```python
from build123d import *

# Parameters (mm, degrees)
SKIZZE1_W                       = 47.557374535
SKIZZE1_H                       = 4
AUFSATZ_LINEAR_AUSTRAGEN1_DEPTH = 76
AUFSATZ_LINEAR_AUSTRAGEN2_DEPTH = 47.557374535
VERRUNDUNG1_R                   = 10
SKIZZE3_R                       = 3.3
SCHNITT_LINEAR_AUSTRAGEN1_DEPTH = 47.557374535
SKIZZE4_W                       = 47.557374535
SKIZZE4_H                       = 15
SCHNITT_LINEAR_AUSTRAGEN2_DEPTH = 30
SKIZZE5_W                       = 47.557374535
SKIZZE5_H                       = 34.5
TEMPOR_R_DEPTH                  = 20


with BuildPart() as part:
    # Skizze1 → Aufsatz-Linear austragen1 (new body)
    with BuildSketch(Plane.ZY.offset(38)):
        with Locations((46.278687268, -2)):
            Rectangle(SKIZZE1_W, SKIZZE1_H)
    extrude(amount=-AUFSATZ_LINEAR_AUSTRAGEN1_DEPTH)

    # Skizze2 → Aufsatz-Linear austragen2 (add)
    with BuildSketch(Plane.XY.offset(22.5)):
        Polygon((-38, 65), (-38, 0), (-28, 0), (-22.226497308, 10), (-28, 20), (-28, 45), (-22.226497308, 55), (-28, 65), align=None)
        Polygon((28, 65), (38, 65), (38, 0), (28, 0), (22.226497308, 10), (28, 20), (28, 45), (22.226497308, 55), align=None)
    extrude(amount=AUFSATZ_LINEAR_AUSTRAGEN2_DEPTH)

    # Verrundung1
    verrundung1_edges = [part.edges().sort_by_distance(p)[0] for p in [
        (-22.226497308, 10, 46.278687268),
        (-22.226497308, 55, 46.278687268),
        (22.226497308, 55, 46.278687268),
        (22.226497308, 10, 46.278687268),
    ]]
    fillet(verrundung1_edges, radius=VERRUNDUNG1_R)

    # Skizze3 → Schnitt-Linear austragen1 (cut)
    with BuildSketch(Plane(origin=(0, 0, 22.5), x_dir=(-1, 0, 0), z_dir=(0, 0, -1))):
        with Locations((32, 10)):
            Circle(SKIZZE3_R)
        with Locations((32, 55)):
            Circle(SKIZZE3_R)
        with Locations((-32, 55)):
            Circle(SKIZZE3_R)
        with Locations((-32, 10)):
            Circle(SKIZZE3_R)
    extrude(amount=-SCHNITT_LINEAR_AUSTRAGEN1_DEPTH, mode=Mode.SUBTRACT)

    # Skizze4 → Schnitt-Linear austragen2 (cut)
    with BuildSketch(Plane.ZY.offset(-38)):
        with Locations((46.278687268, 23)):
            Rectangle(SKIZZE4_W, SKIZZE4_H)
    extrude(amount=SCHNITT_LINEAR_AUSTRAGEN2_DEPTH, mode=Mode.SUBTRACT)


with BuildPart() as schnitt_linear_austragen2_piece_1:
    # of the separate pieces the step leaves, piece 1, a body of its own (schnitt_linear_austragen2_pieces)
    add(part.part.solids().sort_by_distance((38, 15.5, 22.5))[0])


with BuildPart() as schnitt_linear_austragen2_piece_2:
    # of the separate pieces the step leaves, piece 2, a body of its own (schnitt_linear_austragen2_pieces)
    add(part.part.solids().sort_by_distance((25.113248654, 60, 22.5))[0])

    # Skizze5 → temporär (cut)
    with BuildSketch(Plane(origin=(38, 0, 0), x_dir=(0, 0, -1), z_dir=(1, 0, 0))):
        with Locations((-46.278687268, 47.75)):
            Rectangle(SKIZZE5_W, SKIZZE5_H)
    extrude(amount=-TEMPOR_R_DEPTH, mode=Mode.SUBTRACT)


solid = schnitt_linear_austragen2_piece_1.part
```
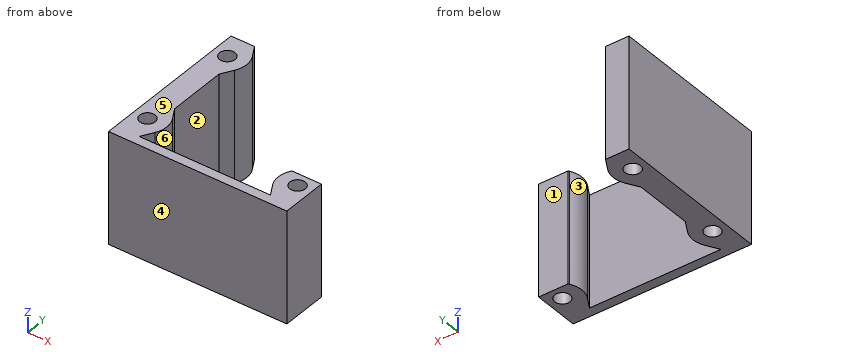
Geometry: final body of the model. Coordinates: model frame, mm. Face numbers are marked on the shaded views. A direction names the side the tool comes from. Round coordinates to 2 decimals unless told otherwise and drop trailing zeros. Write each loop counter-clockwise with the first axis right and the second up, starting at its lowest first coordinate (ties: lowest second). Pieces come first, ordered by that corner, then holes. Notation, with made-up numbers: M -1.75,9.5 L 24.25,9.5 A19 ccw 24.25,38.5 Z; hole C -23,-25.5 d8. An arc over 180 degrees is marked long. Answer in a Markdown table with one row per item. Add a question column.
(1) Cut plane C-C, the plane y = 55. Return the cut outline in (x, z).
(2) Cut plane B-B, the plane z = 28. Return the cut outline in (x, y), then the cut area to 3 significant figures.
(3) Draft query along Y for the marked faces 4, 5 and 6. Return one class per face: pulls with the +Y half, pulls with the -Y half, needs draft (parallel to the pull), parting line crosses it, or undercut.
(4) Reachability of the marked faces 1, 2 and 3 from +Z, -Z, +X, -X, +Y, -Y: full face, straight path, thin tool, end or side. Return the list, or none.
(5) Contact query for flat-ended pins moving along their axis: pin 1 (2 mm diameter, centred on x = 24, y = 15.5, fed in from -Z); pin 2 (5 mm diameter, centred on y = 32.5, z = 46, fed in from +X); pin 3 (1.5 mm diameter, centred on x = 26.5, z = 59.5, fed in from +Y); pin 4 (10 mm diameter, centred on x = -0.5, z = 52.5, fed in from +Y). Output: stop coordinate, or through.
(6) Cut plane A-A, the plane x = -32. Return the cut outline in (y, z), then the cut area to 3 significant figures.
(7) Ray query, L1, parallel to Y at x = -32, z = 41; L2, parallel to Y at x = 32, z = 51.5; L3, parallel to Y at x = -29.5, z = 28. Return the intervals inside material, ascending.
(8) Cut plane D-D, the plane y = 10. Return the cut outline in (x, z).
Established:
| question | item | result |
|---|---|---|
| 1 | outline | M -38,22.5 L -35.3,22.5 L -35.3,70.06 L -38,70.06 Z; M -28.7,22.5 L -23.77,22.5 L -23.77,70.06 L -28.7,70.06 Z |
| 2 | outline | M -38,-4 L 38,-4 L 38,15.5 L 25.4,15.5 L 25.11,15 A10 ccw 25.11,5 L 28,0 L -28,0 L -25.11,5 A10 ccw -25.11,15 L -28,20 L -28,45 L -25.11,50 A10 ccw -25.11,60 L -28,65 L -38,65 Z; hole C -32,10 d6.6; hole C -32,55 d6.6; hole C 32,10 d6.6 |
| 2 | area | 1,160 mm² |
| 3 | face 4 | pulls with the -Y half |
| 3 | face 5 | needs draft |
| 3 | face 6 | undercut |
| 4 | face 1 | +Z, -Z, +X, +Y |
| 4 | face 2 | +Z, -Z, +X |
| 4 | face 3 | +Z, -Z |
| 5 | pin 1 | through |
| 5 | pin 2 | x = -28 |
| 5 | pin 3 | y = 15.5 |
| 5 | pin 4 | y = 0 |
| 6 | outline | M -4,22.5 L 6.7,22.5 L 6.7,70.06 L -4,70.06 Z; M 13.3,22.5 L 51.7,22.5 L 51.7,70.06 L 13.3,70.06 Z; M 58.3,22.5 L 65,22.5 L 65,70.06 L 58.3,70.06 Z |
| 6 | area | 2,650 mm² |
| 7 | L1 | -4 to 6.7, 13.3 to 51.7, 58.3 to 65 |
| 7 | L2 | -4 to 6.7, 13.3 to 15.5 |
| 7 | L3 | -4 to 7.85, 12.15 to 52.85, 57.15 to 65 |
| 8 | outline | M -38,22.5 L -35.3,22.5 L -35.3,70.06 L -38,70.06 Z; M -28.7,22.5 L -23.77,22.5 L -23.77,70.06 L -28.7,70.06 Z; M 23.77,22.5 L 28.7,22.5 L 28.7,70.06 L 23.77,70.06 Z; M 35.3,22.5 L 38,22.5 L 38,70.06 L 35.3,70.06 Z |
